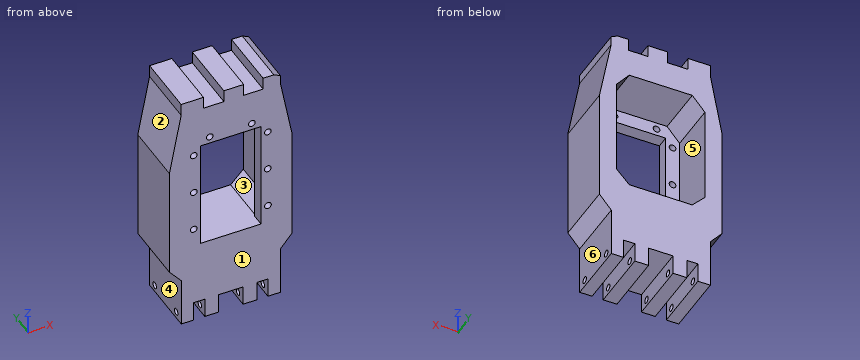
```python
from build123d import *

# Parameters (mm, degrees)
SZKIC1_R                    = 1.35
SZKIC1_W                    = 24.4
SZKIC1_H                    = 45
DODANIE_WYCI_GNI_CIE1_DEPTH = 5
DODANIE_WYCI_GNI_CIE2_DEPTH = 25
SZKIC8_W                    = 8
SZKIC8_H                    = 5
SZKIC8_W_2                  = 9
DODANIE_WYCI_GNI_CIE3_DEPTH = 25
SZKIC7_R                    = 1.35
WYTNIJ_WYCI_GNI_CIE8_DEPTH  = 45.8


with BuildPart() as part:
    # Szkic1 → Dodanie-wyci_gni_cie1 (new body)
    with BuildSketch(Plane(origin=(0, 0, 0), x_dir=(1, 0, 0), z_dir=(0, 1, 0))):
        Polygon((10.047789553, 143.7963255), (14.547789553, 143.7963255), (14.547789553, 151.7963255), (19.547789553, 151.7963255), (19.547789553, 131.76713902), (24.347789553, 126.117958863), (24.347789553, 80.533497461), (19.595579106, 55.3963255), (-20.5, 55.3963255), (-25.252210447, 80.533497461), (-25.252210447, 126.117958863), (-20.452210447, 131.76713902), (-20.452210447, 151.7963255), (-15.452210447, 151.7963255), (-15.452210447, 143.7963255), (-10.952210447, 143.7963255), (-10.952210447, 151.7963255), (-5.399500142, 151.7963255), (-5.399500142, 143.7963255), (4.495079248, 143.7963255), (4.495079248, 151.7963255), (10.047789553, 151.7963255), align=None)
        with Locations((14.547789553, 109.8963255)):
            Circle(SZKIC1_R, mode=Mode.SUBTRACT)
        with Locations((14.5, 92.8963255)):
            Circle(SZKIC1_R, mode=Mode.SUBTRACT)
        with Locations((14.5, 75.8963255)):
            Circle(SZKIC1_R, mode=Mode.SUBTRACT)
        with Locations((8.047789553, 69.5963255)):
            Circle(SZKIC1_R, mode=Mode.SUBTRACT)
        with Locations((-8.952210447, 69.5963255)):
            Circle(SZKIC1_R, mode=Mode.SUBTRACT)
        with Locations((-15.404420894, 75.8963255)):
            Circle(SZKIC1_R, mode=Mode.SUBTRACT)
        with Locations((-15.404420894, 92.8963255)):
            Circle(SZKIC1_R, mode=Mode.SUBTRACT)
        with Locations((-15.452210447, 109.8963255)):
            Circle(SZKIC1_R, mode=Mode.SUBTRACT)
        with Locations((-0.452210447, 94.8963255)):
            Rectangle(SZKIC1_W, SZKIC1_H, mode=Mode.SUBTRACT)
    extrude(amount=DODANIE_WYCI_GNI_CIE1_DEPTH)

    # Szkic1_3 → Dodanie-wyci_gni_cie2 (add)
    with BuildSketch(Plane(origin=(0, 0, 0), x_dir=(1, 0, 0), z_dir=(0, 1, 0))):
        Polygon((14.547789553, 143.7963255), (10.047789553, 143.7963255), (10.047789553, 151.7963255), (4.495079248, 151.7963255), (4.495079248, 143.7963255), (-5.399500142, 143.7963255), (-5.399500142, 151.7963255), (-10.952210447, 151.7963255), (-10.952210447, 143.7963255), (-15.452210447, 143.7963255), (-15.452210447, 151.7963255), (-20.452210447, 151.7963255), (-20.452210447, 131.76713902), (-25.252210447, 126.117958863), (-25.252210447, 80.533497461), (-20.5, 55.3963255), (19.595579106, 55.3963255), (24.347789553, 80.533497461), (24.347789553, 126.117958863), (19.547789553, 131.76713902), (19.547789553, 151.7963255), (14.547789553, 151.7963255), align=None)
        Polygon((-13.152210447, 117.3963255), (-12.652210447, 117.3963255), (11.747789553, 117.3963255), (12.247789553, 117.3963255), (17.347789553, 112.070622628), (17.347789553, 72.740102496), (12.295579106, 66.7963255), (-13.2, 66.7963255), (-18.252210447, 72.740102496), (-18.252210447, 112.070622628), align=None, mode=Mode.SUBTRACT)
    extrude(amount=DODANIE_WYCI_GNI_CIE2_DEPTH)

    # Szkic8 → Dodanie-wyci_gni_cie3 (add)
    with BuildSketch(Plane(origin=(0, 25, 0), x_dir=(1, 0, 0), z_dir=(0, 1, 0))):
        Polygon((19.595579106, 51.744454691), (19.595579106, 55.3963255), (12.595579106, 55.3963255), (12.595579106, 50.3963255), (16.925579106, 50.3963255), align=None)
        with Locations((0.758846465, 52.8963255)):
            Rectangle(SZKIC8_W, SZKIC8_H)
        with Locations((-16, 52.8963255)):
            Rectangle(SZKIC8_W_2, SZKIC8_H)
    extrude(amount=-DODANIE_WYCI_GNI_CIE3_DEPTH)

    # Szkic7 → Wytnij-wyci_gni_cie8 (cut, through all)
    with BuildSketch(Plane.ZY.offset(20.452210447)):
        with Locations((-148.9963255, 21)):
            Circle(SZKIC7_R)
        with Locations((-148.9963255, 4)):
            Circle(SZKIC7_R)
    extrude(amount=-WYTNIJ_WYCI_GNI_CIE8_DEPTH, mode=Mode.SUBTRACT)


solid = part.part
```
For this review, take the finished solid that the model builds, in its own axes (mm). Face numbers are marked on the shaded views. A direction names the side the tool comes from. Coordinates: 2 decimals unless noted, no trailing zeros. Write each loop counter-clockwise with the first axis right and the second up, starting at its lowest first coordinate (ties: lowest second). Pieces come first, ordered by that corner, then holes. Notation, with made-up numbers: (-37.75, -32.5) - (-2.75, -32.5) arc R7 ccw to (-2.75, -19.5) - close; hole circle Ø2 at (71.5, -10.5). An arc over 180 degrees is marked (long way). Answer in a Markdown table with one row per item. Add a question column.
Q1. We need section B-B, the plane z = -96.5. State the section outline as (x, y) points, and give its area (3 significant figures).
Q2. Tool access review of the marked faces 4, 5 and 6: name each direction out of +Z, -Z, +X, -X, +Y, -Y from which nothing blocks a thin tool from reaching the whole face with its end or side.
Q3. For probe 1 along X at (y, z) = (12.75, -55); probe 2 along X at (y, z) = (7, -90); probe 3 along Z at (x, y) = (3, 23.5), list the stretches that pass through material, from the lowest coordinate up.
Q4. We need section A-A, the plane x = -2. State the section outline as (y, z) points, and give its area (3 significant figures).
Q5. Draft analysis for pull direction X (two halves, no side actions). For the marked faces 1, 2 and 3, state which applies: +X half, -X half, draft (parallel to the pull), parting line (faces both ways), or undercut.
Q6. For P1, Ø2.5, axis at x = 8.05, z = -69.6, coming from the +Y side; P2, Ø6, axis at y = 20.5, z = -72.5, coming from the -X side; P3, Ø4.5, axis at y = 21, z = -149, coming from the +X side; P4, Ø1.5, axis at y = 11, z = -53, coming from the +X side, all flat-tipped, find the tip position at first contact; note any pin that passes through.
Q7. We need section C-C, the plane y = 21. Count the separate pieces of the cut face and the enclosed holes in it, and give its area (3 significant figures).
Answer list:
| question | item | result |
|---|---|---|
| 1 | outline | (-25.25, 0) - (-12.65, 0) - (-12.65, 5) - (-18.25, 5) - (-18.25, 25) - (-25.25, 25) - close; (11.75, 0) - (24.35, 0) - (24.35, 25) - (17.35, 25) - (17.35, 5) - (11.75, 5) - close |
| 1 | area | 406 mm2 |
| 2 | face 4 | -Z, -X, +Y, -Y |
| 2 | face 5 | +Y |
| 2 | face 6 | -Z, +X, +Y, -Y |
| 3 | probe 1 | x = -20.5 to -11.5, -3.24 to 4.76, 12.6 to 19.6 |
| 3 | probe 2 | x = -25.25 to -18.25, 17.35 to 24.35 |
| 3 | probe 3 | z = -143.8 to -117.4, -66.8 to -50.4 |
| 4 | outline | (0, -143.8) - (25, -143.8) - (25, -117.4) - (0, -117.4) - close; (0, -72.4) - (5, -72.4) - (5, -66.8) - (25, -66.8) - (25, -50.4) - (0, -50.4) - close |
| 4 | area | 1,100 mm2 |
| 5 | face 1 | draft |
| 5 | face 2 | -X half |
| 5 | face 3 | undercut |
| 6 | P1 | passes through |
| 6 | P2 | stops at x = -24.3 |
| 6 | P3 | stops at x = 19.55 |
| 6 | P4 | stops at x = 19.6 |
| 7 | separate pieces | 5 |
| 7 | enclosed holes | 1 |
| 7 | area | 2,610 mm2 |
